The drawing under review shows one solid part. Ordinate dimensions are in mm from its lowest x, y, z. Give positions to 0.01 mm unless a question says otherwise; leave off trailing zeros. Loops run counter-clockwise (first coordinate to the right, second up) from the corner with the lowest first, then second, coordinate; pieces in that order, holes last. Notation, with made-up numbers: (75.5, 57) -> (127.5, 57) arc R15 cw to (127.5, 75) -> close; hole circle Ø11 at (-6, -22.5). An arc over 180 degrees is marked (long way). Answer in a Markdown table with one row per item. Add a question column.
(1) Consider section D-D on z = 3.5. Write out the cut boundary in (x, y), then the cut area to 3 significant figures.
(2) Consider section B-B on x = 3.5. Write out the cut boundary in (y, z), then the cut area to 3 significant figures.
(3) Consider section A-A on z = 33.5. Write out the cut boundary in (x, y).
(4) For pin 1 (4 mm diameter, centred on x = 32.5, z = 31, fed in from +Y); pin 2 (1.5 mm diameter, centred on y = 3, z = 3.5, fed in from +X); pin 3 (1.5 mm diameter, centred on x = 28, y = 4, fed in from +Z), all flat-tipped, find the tip position at first contact; note any pin that passes through.
(5) Consider section C-C on x = 9. Write out the cut boundary in (y, z), then the cut area to 3 significant figures.
(6) For line 1 (Z direction, x = 3.5, y = 1.15); line 2 (X direction, y = 0.95, z = 33.5); line 3 (Y direction, x = 14.5, z = 26.5), list the stretches that pass through material, from the lowest coordinate up.
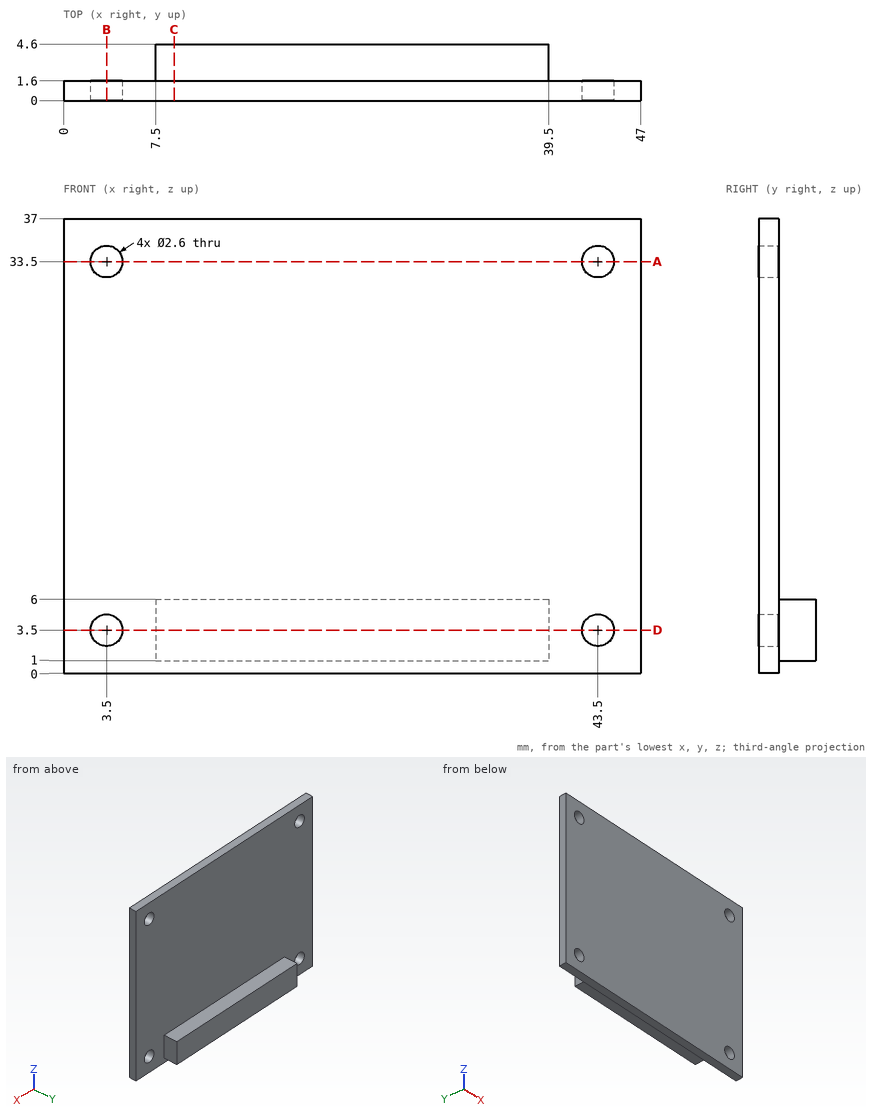
Values follow:
| question | item | result |
|---|---|---|
| 1 | outline | (0, 0) -> (2.2, 0) -> (2.2, 1.6) -> (0, 1.6) -> close; (4.8, 0) -> (42.2, 0) -> (42.2, 1.6) -> (39.5, 1.6) -> (39.5, 4.6) -> (7.5, 4.6) -> (7.5, 1.6) -> (4.8, 1.6) -> close; (44.8, 0) -> (47, 0) -> (47, 1.6) -> (44.8, 1.6) -> close |
| 1 | area | 163 mm2 |
| 2 | outline | (0, 0) -> (1.6, 0) -> (1.6, 2.2) -> (0, 2.2) -> close; (0, 4.8) -> (1.6, 4.8) -> (1.6, 32.2) -> (0, 32.2) -> close; (0, 34.8) -> (1.6, 34.8) -> (1.6, 37) -> (0, 37) -> close |
| 2 | area | 50.9 mm2 |
| 3 | outline | (0, 0) -> (2.2, 0) -> (2.2, 1.6) -> (0, 1.6) -> close; (4.8, 0) -> (42.2, 0) -> (42.2, 1.6) -> (4.8, 1.6) -> close; (44.8, 0) -> (47, 0) -> (47, 1.6) -> (44.8, 1.6) -> close |
| 4 | pin 1 | y = 1.6 |
| 4 | pin 2 | x = 39.5 |
| 4 | pin 3 | z = 6 |
| 5 | outline | (0, 0) -> (1.6, 0) -> (1.6, 1) -> (4.6, 1) -> (4.6, 6) -> (1.6, 6) -> (1.6, 37) -> (0, 37) -> close |
| 5 | area | 74.2 mm2 |
| 6 | line 1 | 0 to 2.2, 4.8 to 32.2, 34.8 to 37 |
| 6 | line 2 | 0 to 2.2, 4.8 to 42.2, 44.8 to 47 |
| 6 | line 3 | 0 to 1.6 |
